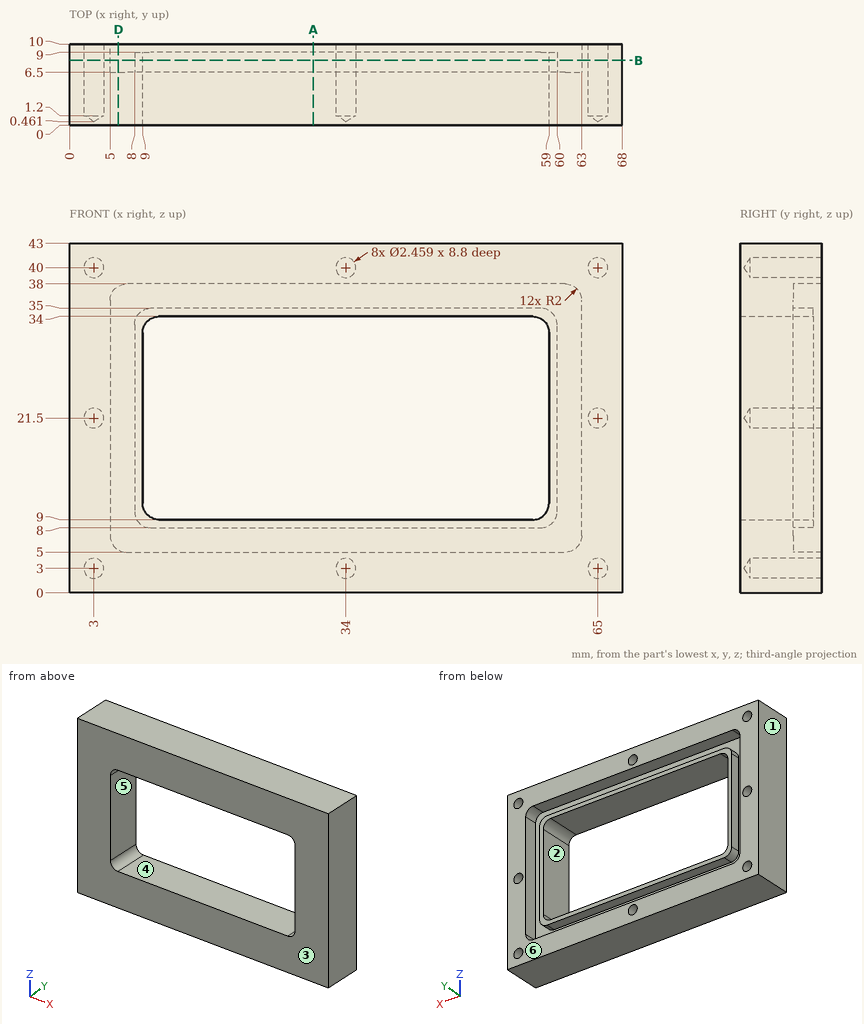
Answer from the drawing. Dimensions are ordinates in mm from the lowest x, y and z of the part. A direction names the side the tool comes from. Round coordinates to 2 decimals unless told otherwise and drop trailing zeros. Write each loop counter-clockwise with the first axis right and the second up, starting at its lowest first coordinate (ties: lowest second). Pieces come first, ordered by that corner, then holes.
1. Which of the six approach directions +Z, -Z, +X, -X, +Y, -Y give full straight-line access (tool end or side, diameter ignored) to the marked faces 5 and 6?
2. The part is cut by section B-B, the plane y = 8. State how many separate pieces and enclosed holes the cut face has, then the cut area to 3 significant figures.
3. Determine the mould class of the marked faces 1, 2, 3 and 4 for opening direction X: pulls with the +X half, pulls with the -X half, needs draft (parallel to the pull), parting line crosses it, or undercut.
4. Given pin 1 Ø2 at (x, z) = (3, 40) entering from +Y; pin 2 Ø13.5 at (x, z) = (43, 27.5) entering from +Y, each flat-ended and moving along its own axis, determine where each tip first touches the part or whether it passes through.
5. Straight lines are drawn through the part: L1, parallel to Z at x = 3, y = 7.5; L2, parallel to X at y = 6, z = 40; L3, parallel to X at y = 4, z = 21.5. For each, find the intervals that lie inside material, in ascending order.
6. The part is cut by section A-A, the plane x = 30. Determine the outline of the cut face in (y, z), then the cut area to 3 significant figures.
7. The part is cut by section D-D, the plane x = 6. Determine the outline of the cut face in (y, z).
Values:
1. face 5: +Y, -Y
1. face 6: +Z, -Z, +X, -X, +Y
2. separate pieces: 2
2. enclosed holes: 10
2. area: 1,130 mm2
3. face 1: pulls with the -X half
3. face 2: undercut
3. face 3: needs draft
3. face 4: undercut
4. pin 1: stops at y = 1.06
4. pin 2: stops at y = 9
5. L1: z = 0 to 1.77, 4.23 to 20.27, 22.73 to 38.77, 41.23 to 43
5. L2: x = 0 to 1.77, 4.23 to 32.77, 35.23 to 63.77, 66.23 to 68
5. L3: x = 0 to 1.77, 4.23 to 9, 59 to 63.77, 66.23 to 68
6. outline: (0, 0) - (10, 0) - (10, 5) - (6.5, 5) - (6.5, 8) - (9, 8) - (9, 9) - (0, 9) - close; (0, 34) - (9, 34) - (9, 35) - (6.5, 35) - (6.5, 38) - (10, 38) - (10, 43) - (0, 43) - close
6. area: 157 mm2
7. outline: (0, 0) - (10, 0) - (10, 5.27) - (6.5, 5.27) - (6.5, 37.73) - (10, 37.73) - (10, 43) - (0, 43) - close
